Source: three-view drawing plus pictorial views. Frame: mm from the lowest corner of the part. A direction names the side the tool comes from. Coordinates: 2 decimals unless noted, no trailing zeros. Loops run counter-clockwise (first coordinate to the right, second up) from the corner with the lowest first, then second, coordinate; pieces in that order, holes last. Notation, with made-up numbers: (32.25, 12) - (37.25, 12) arc R17 cw to (37.25, 32) - close; hole circle Ø10 at (40.5, 86). An arc over 180 degrees is marked (long way). Answer as CSV lines item,"result". Start each with the question number.
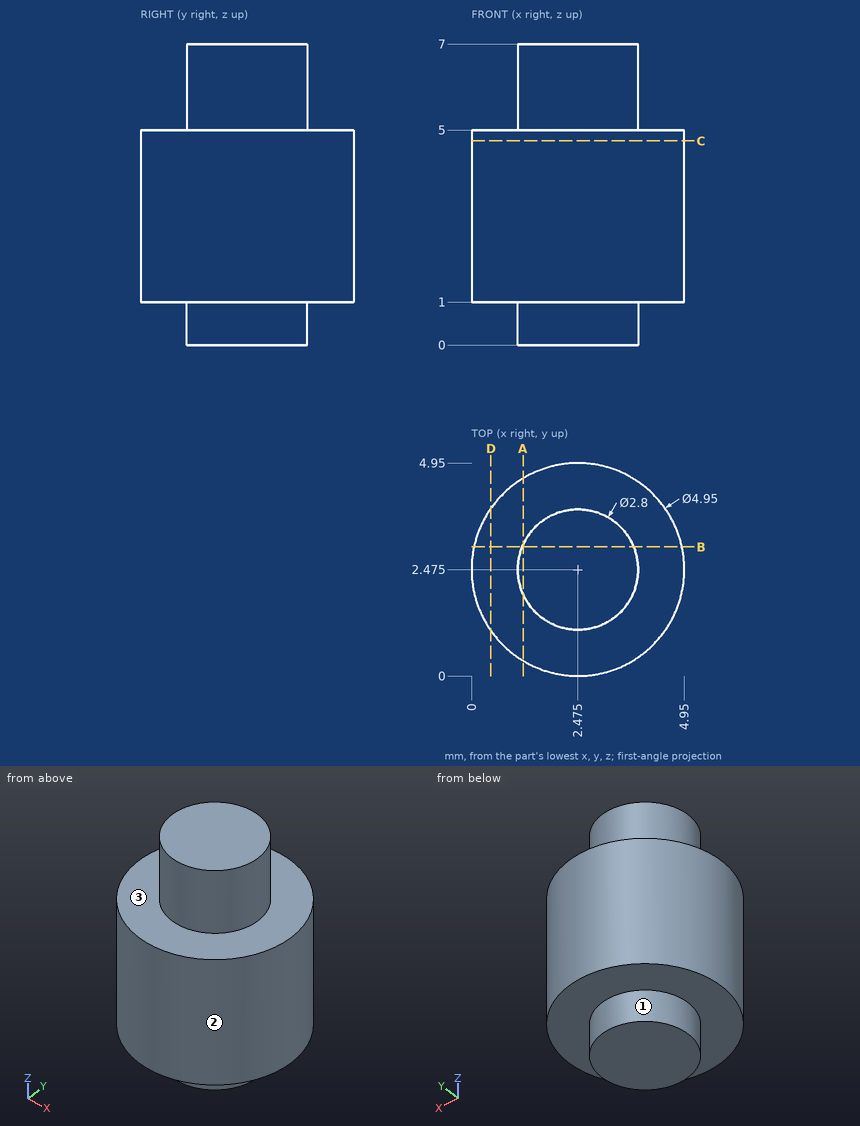
Item 1: Section query B-B, the plane y = 3. Output: boundary loops of the cut face in (x, z).
Item 2: Section query D-D, the plane x = 0.45. Output: boundary loops of the cut face in (y, z), and give its area (3 significant figures).
Item 3: Contact query for a flat-ended pin moving along its axis: P1, Ø1.5, axis at x = 0.5, y = 3, coming from the -Z side. Output: stop coordinate, or through.
Item 4: Section query A-A, the plane x = 1.2. Output: boundary loops of the cut face in (y, z).
Item 5: Section query C-C, the plane z = 4.75. Output: boundary loops of the cut face in (x, y) (3 decimals), and give its area (3 significant figures).
Item 6: Material intervals for probe 1 along Z at (x, y) = (0.5, 2.35); probe 2 along X at (y, z) = (2.4, 2.5); probe 3 along Y at (x, z) = (0.6, 3.5), sorted ascending.
Item 7: Set-up query: the marked faces 1, 2 and 3. Return all of +Z, -Z, +X, -X, +Y, -Y with unobstructed straight access to the full face (end or side cutting, diameter ignored); none if empty.
Response values:
1,outline,"(0.06, 1) - (1.18, 1) - (1.18, 0) - (3.77, 0) - (3.77, 1) - (4.89, 1) - (4.89, 5) - (3.77, 5) - (3.77, 7) - (1.18, 7) - (1.18, 5) - (0.06, 5) - close"
2,outline,"(1.05, 1) - (3.9, 1) - (3.9, 5) - (1.05, 5) - close"
2,area,"11.4 mm²"
3,P1,"stops at z = 0"
4,outline,"(0.35, 1) - (1.9, 1) - (1.9, 0) - (3.05, 0) - (3.05, 1) - (4.6, 1) - (4.6, 5) - (3.05, 5) - (3.05, 7) - (1.9, 7) - (1.9, 5) - (0.35, 5) - close"
5,outline,"circle Ø4.95 at (2.475, 2.475)"
5,area,"19.2 mm²"
6,probe 1,"z = 1 to 5"
6,probe 2,"x = 0 to 4.95"
6,probe 3,"y = 0.86 to 4.09"
7,face 1,"-Z"
7,face 2,"+Z, -Z"
7,face 3,"+Z"
